The figure shows three views and two pictorial views of one solid part (mm, origin at its lowest corner). Answer the questions. Give positions to 0.01 mm unless a question says otherwise; leave off trailing zeros. Order: outer loops, then holes, each group sorted by start corner. A loop starts at its lowest first (then second) coordinate and runs counter-clockwise, first axis right, second up. Notation, with made-up numbers: (59, 14) - (69, 14) arc R13 cw to (69, 18) - close; hole circle Ø4 at (73.5, 54). An arc over 180 degrees is marked (long way). Use a Markdown table: item, result. Add a question column.
1. For a pull along X with two mould halves and no side action, classify the marked faces 1, 2, 3 and 4 as released by +X, released by -X, zero draft, split by the parting line, or undercut.
2. Consider L1, parallel to X at y = 8.75, z = 2.7; L2, parallel to Y at x = 62, z = 1.65; L3, parallel to X at y = 5, z = 3.1. Determine where each line is inside the solid, lowest interval first.
3. A cutting plane is placed at B-B on z = 1.8. Determine the outline of the cut face in (x, y).
4. A cutting plane is placed at C-C on y = 16. Determine the outline of the cut face in (x, z).
5. Flat-ended cylindrical pins translate along their axes: P1, Ø9.5, axis at x = 114, y = 9, coming from the -Z side; P2, Ø2, axis at y = 14, z = 1, coming from the -X side; P3, Ø3, axis at y = 6.5, z = 3.5, coming from the -X side; P4, Ø5, axis at x = 65.5, y = 10.5, coming from the -Z side. Find the tip coordinate at first contact, or state that the pin passes through.
6. A cutting plane is placed at A-A on x = 40. Determine the outline of the cut face in (y, z), and give its area (3 significant figures).
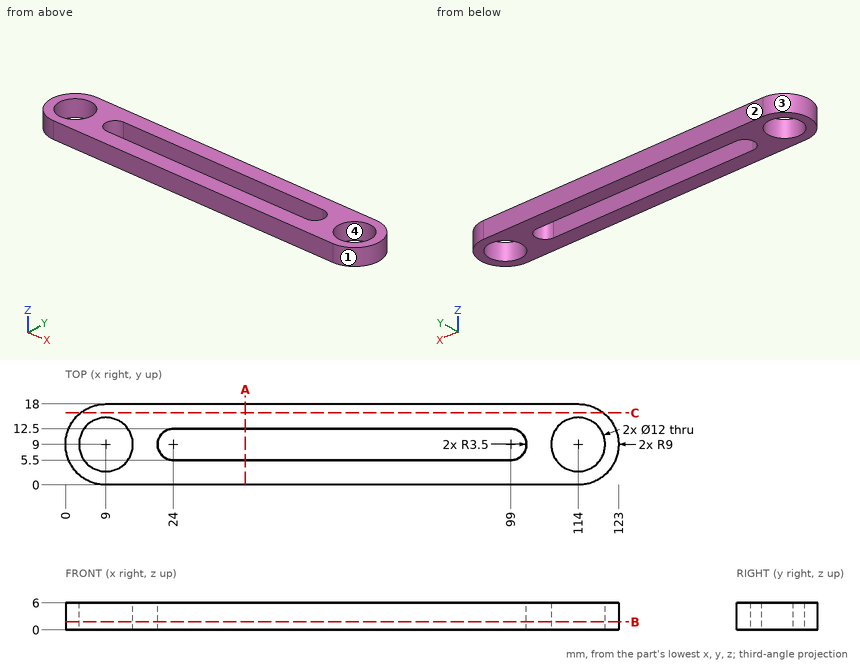
Output values:
| question | item | result |
|---|---|---|
| 1 | face 1 | released by +X |
| 1 | face 2 | zero draft |
| 1 | face 3 | released by -X |
| 1 | face 4 | undercut |
| 2 | L1 | 0 to 3.01, 14.99 to 20.51, 102.49 to 108.01, 119.99 to 123 |
| 2 | L2 | 0 to 5.5, 12.5 to 18 |
| 2 | L3 | 0.94 to 4.53, 13.47 to 109.53, 118.47 to 122.06 |
| 3 | outline | (9, 0) - (114, 0) arc R9 ccw to (114, 18) - (9, 18) arc R9 ccw to start; hole circle Ø12 at (9, 9); hole (24, 5.5) - (99, 5.5) arc R3.5 ccw to (99, 12.5) - (24, 12.5) arc R3.5 ccw to start; hole circle Ø12 at (114, 9) |
| 4 | outline | (3.34, 0) - (119.66, 0) - (119.66, 6) - (3.34, 6) - close |
| 5 | P1 | through |
| 5 | P2 | x = 0.94 |
| 5 | P3 | x = 0.06 |
| 5 | P4 | z = 0 |
| 6 | outline | (0, 0) - (5.5, 0) - (5.5, 6) - (0, 6) - close; (12.5, 0) - (18, 0) - (18, 6) - (12.5, 6) - close |
| 6 | area | 66.0 mm² |
